```python
from build123d import *

# Parameters (mm, degrees)
F0_W     = 50.8
F0_H     = 12.7
F0_H_2   = 25.4
F1_DEPTH = 38.1
F0_W_2   = 25.4
F2_DEPTH = 50.8
F5_DEPTH = 63.5
F4_W     = 25.4
F4_H     = 25.4
F6_DEPTH = 88.9
F8_DEPTH = 25.4


with BuildPart() as f1:
    # F0 (on Top) → F1 (new body)
    with BuildSketch(Plane.XY):
        with Locations((0, -25.4)):
            Rectangle(F0_W, F0_H)
        with Locations((0, -6.35)):
            Rectangle(F0_W, F0_H_2)
        with Locations((0, 19.05)):
            Rectangle(F0_W, F0_H_2)
    extrude(amount=F1_DEPTH)

    # F0 (on Top) → F2 (join)
    with BuildSketch(Plane.XY):
        with Locations((-38.1, 19.05)):
            Rectangle(F0_W_2, F0_H_2)
        with Locations((-38.1, -6.35)):
            Rectangle(F0_W_2, F0_H_2)
        with Locations((-38.1, -25.4)):
            Rectangle(F0_W_2, F0_H)
    extrude(amount=F2_DEPTH)

    # F3 (on face) → F5 (join)
    with BuildSketch(Plane.XZ.offset(31.75)):
        Polygon((50.8, 0), (25.4, 38.1), (25.4, 0), align=None)
    extrude(amount=-F5_DEPTH)

    # F4 (on face) → F6 (cut, symmetric)
    with BuildSketch(Plane.YZ.offset(25.4)):
        with Locations((-6.35, 12.7)):
            Rectangle(F4_W, F4_H)
    extrude(amount=F6_DEPTH, both=True, mode=Mode.SUBTRACT)

    # F7 (on face) → F8 (join)
    with BuildSketch(Plane(origin=(-50.8, 0, 0), x_dir=(0, -1, 0), z_dir=(-1, 0, 0))):
        with BuildLine():
            Line((15.6470452561, 50.8), (19.05, 50.8))
            Line((19.05, 50.8), (31.75, 50.8))
            Line((31.75, 50.8), (15.1117039467, 77.08511184))
            ThreePointArc((15.1117039467, 77.08511184), (18.0455659931, 70.5722245353), (19.05, 63.5))
            ThreePointArc((19.05, 63.5), (18.1845159877, 56.9259962544), (15.6470452561, 50.8))
        make_face()
        with BuildLine():
            Line((-6.3500000221, 50.8), (15.6470452561, 50.8))
            ThreePointArc((15.6470452561, 50.8), (18.1845159877, 56.9259962544), (19.05, 63.5))
            ThreePointArc((19.05, 63.5), (18.0455659931, 70.5722245353), (15.1117039467, 77.08511184))
            ThreePointArc((15.1117039467, 77.08511184), (-13.4222245353, 87.8955659931), (-31.75, 63.5))
            ThreePointArc((-31.75, 63.5), (-30.8845159877, 56.9259962544), (-28.3470452561, 50.8))
            Line((-28.3470452561, 50.8), (-6.3500000221, 50.8))
        make_face()
        with BuildLine():
            ThreePointArc((6.35, 63.5), (2.6302561133, 54.5197438711), (-6.3500000221, 50.8))
            ThreePointArc((-6.3500000221, 50.8), (-15.3302561133, 72.4802561289), (6.35, 63.5))
        make_face(mode=Mode.SUBTRACT)
        with BuildLine():
            ThreePointArc((-28.3470452561, 50.8), (-6.35, 38.1), (15.6470452561, 50.8))
            Line((15.6470452561, 50.8), (-6.3500000221, 50.8))
            Line((-6.3500000221, 50.8), (-28.3470452561, 50.8))
        make_face()
        with BuildLine():
            Line((-31.75, 50.8), (-28.3470452561, 50.8))
            ThreePointArc((-28.3470452561, 50.8), (-30.8845159877, 56.9259962544), (-31.75, 63.5))
            Line((-31.75, 63.5), (-31.75, 50.8))
        make_face()
    extrude(amount=-F8_DEPTH)


solid = f1.part
```
For this review, take the finished solid that the model builds, in its own axes (mm). A direction names the side the tool comes from. Coordinates: 2 decimals unless noted, no trailing zeros. Write each loop counter-clockwise with the first axis right and the second up, starting at its lowest first coordinate (ties: lowest second). Pieces come first, ordered by that corner, then holes. Notation, with made-up numbers: (13, -32.5) - (30, -32.5) arc R12 ccw to (30, -21.5) - close; hole circle Ø8 at (8, 12.25). An arc over 180 degrees is marked (long way). Answer in a Markdown table with one row per item. Add a question column.
Q1. Draft analysis for pull direction Y (two halves, no side actions). For faces 1 (the cylindrical face through (-38.28, 12.98, 88.02)), 2 (the flat face through (-12, -31.75, 20)), 3 (the flat face through (-25.4, 0, 52)), 4 (the flat face through (-8, -7, 25.4)), state which applies: +Y half, -Y half, draft (parallel to the pull), parting line (faces both ways), or undercut.
Q2. For probe 1 along Y at (x, z) = (-7, 16.5); probe 2 along Z at (x, y) = (-32, 6); probe 3 along Z at (x, y) = (-46, 12.5), list the stretches that pass through material, from the lowest coordinate up.
Q3. We need section B-B, the plane x = 15. State the section outline as (y, z) points, and give its area (3 significant figures).
Q4. Tool access review of faces 5 (the flat face through (0, 0, 38.1)), 6 (the flat face through (-1, 19, 0)), 7 (the flat face through (1, -19.05, 13)): name each direction out of +Z, -Z, +X, -X, +Y, -Y from which nothing blocks a thin tool from reaching the whole face with its end or side.
Q5. For P1, Ø3, axis at y = -17.5, z = 45.5, coming from the +X side; P2, Ø7.5, axis at x = -29, y = -7.5, coming from the -Z side, all flat-tipped, find the tip position at first contact; note any pin that passes through.
Q6. We need section A-A, the plane x = 36.5. State the section outline as (y, z) points.
Q7. We need section D-D, the plane z = 46.5. State the section outline as (x, y) points.
Q8. We need section C-C, the plane y = -2. State the section outline as (x, z) points, and give its area (3 significant figures).
Answer list:
| question | item | result |
|---|---|---|
| 1 | face 1 | parting line |
| 1 | face 2 | -Y half |
| 1 | face 3 | draft |
| 1 | face 4 | undercut |
| 2 | probe 1 | y = -31.75 to -19.05, 6.35 to 31.75 |
| 2 | probe 2 | z = 25.4 to 50.8, 76.2 to 88.9 |
| 2 | probe 3 | z = 0 to 52.39, 74.61 to 88.14 |
| 3 | outline | (-31.75, 0) - (-19.05, 0) - (-19.05, 25.4) - (6.35, 25.4) - (6.35, 0) - (31.75, 0) - (31.75, 38.1) - (-31.75, 38.1) - close |
| 3 | area | 1,770 mm2 |
| 4 | face 5 | +Z, +X, +Y, -Y |
| 4 | face 6 | -Z, +X, -X, +Y, -Y |
| 4 | face 7 | -Z, +X, -X |
| 5 | P1 | stops at x = -25.4 |
| 5 | P2 | stops at z = 25.4 |
| 6 | outline | (-31.75, 0) - (-19.05, 0) - (-19.05, 21.45) - (-31.75, 21.45) - close; (6.35, 0) - (31.75, 0) - (31.75, 21.45) - (6.35, 21.45) - close |
| 7 | outline | (-50.8, -31.75) - (-25.4, -31.75) - (-25.4, 31.75) - (-50.8, 31.75) - close |
| 8 | outline | (-50.8, 25.4) - (33.87, 25.4) - (25.4, 38.1) - (-25.4, 38.1) - (-25.4, 53.93) - (-50.8, 53.93) - close; (-50.8, 73.07) - (-25.4, 73.07) - (-25.4, 87.49) - (-50.8, 87.49) - close |
| 8 | area | 1,790 mm2 |
